Here's how the part is built. I have some questions about the finished solid (model axes, mm). Face numbers are marked on the shaded views. A direction names the side the tool comes from. Round coordinates to 2 decimals unless told otherwise and drop trailing zeros. Write each loop counter-clockwise with the first axis right and the second up, starting at its lowest first coordinate (ties: lowest second). Pieces come first, ordered by that corner, then holes. Notation, with made-up numbers: (-37.75, -1.5) -> (-14.75, -1.5) arc R29 ccw to (-14.75, 18.5) -> close; hole circle Ø9 at (68, 35). An arc over 180 degrees is marked (long way). Put each result on its own line as item: value. Start each with the question number.
1. Suppose I cut it at B-B (z = 25). Count the separate pieces of the cut face and the enclosed holes in it, then the cut area to 3 significant figures.
2. Suppose I cut it at A-A (y = 47.5). Please give me the cut outline in (x, z).
3. We'd pull the mould along Y, two halves only. Please class the marked faces 1, 2, 3 and 4: +Y half, -Y half, draft (parallel to the pull), parting line (faces both ways), or undercut.
4. I need wall thicknesses on probe 1 along Y at (x, z) = (0, 21); probe 2 along Y at (x, z) = (0, -3); probe 3 along Z at (x, y) = (-28, 38). Which ranges of each line are inside material? Lowest first, please. Write a range as from..to.
5. For pin 1 (8 mm diameter, centred on x = 25, y = 65, fed in from -Z); pin 2 (3 mm diameter, centred on y = 13, z = 49.5, fed in from +X); pin 3 (7 mm diameter, centred on x = 0, y = 0, fed in from -Z); pin 4 (6 mm diameter, centred on x = -58, y = 32, fed in from -Z), each with a flat end and sliding along its axis, tell me the tip position at first contact or that it passes through.
6. Suppose I cut it at D-D (y = 31). Please give me the cut outline in (x, z), then the cut area to 3 significant figures.
7. Which directions (+Z, -Z, +X, -X, +Y, -Y) give clear straight access to the entire face, cutting with the end or side of a thin tool? Please do the marked faces 5, 6, 7 and 8.
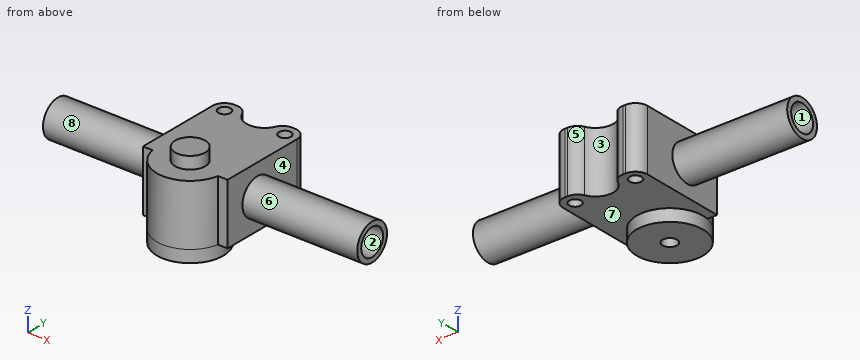
```python
from build123d import *

# Parameters (mm, degrees)
SKETCH1_R           = 5
BOSS_EXTRUDE2_DEPTH = 50
SHELL2_START        = 5
SHELL2_DEPTH        = 40
SKETCH3_R           = 15
CUT_EXTRUDE1_DEPTH  = 5
BOSS_EXTRUDE3_START = 10
SKETCH4_R           = 27.5
SKETCH4_R_2         = 6
BOSS_EXTRUDE3_DEPTH = 10
SKETCH5_R           = 15
SKETCH5_R_2         = 11
BOSS_EXTRUDE4_DEPTH = 95
CUT_EXTRUDE2_START  = -80
SKETCH5_2_R         = 11
CUT_EXTRUDE2_DEPTH  = 80
BOSS_EXTRUDE5_START = -165
SKETCH5_3_R         = 15
SKETCH5_3_R_2       = 11
BOSS_EXTRUDE5_DEPTH = 95
SKETCH6_R           = 12.5
SKETCH6_R_2         = 6
BOSS_EXTRUDE6_DEPTH = 5
CUT_EXTRUDE3_START  = -5
SKETCH6_2_R         = 6
CUT_EXTRUDE3_DEPTH  = 5
BOSS_EXTRUDE7_START = -38
SKETCH6_3_R         = 12.5
SKETCH6_3_R_2       = 6
BOSS_EXTRUDE7_DEPTH = 38
SKETCH6_4_R         = 12.5
SKETCH6_4_R_2       = 6
BOSS_EXTRUDE8_DEPTH = 10


# Read off the part's stored shape, not the designer's step: Shell2
with BuildPart() as part:
    # Sketch1 → Boss-Extrude2 (new body)
    with BuildSketch(Plane.XY):
        with BuildLine():
            Line((22.912878475, 75), (25, 75))
            ThreePointArc((25, 75), (32.071067812, 72.071067812), (35, 65))
            Line((35, 65), (35, -5))
            Line((35, -5), (27.041634566, -5))
            ThreePointArc((27.041634566, -5), (0, -27.5), (-27.041634566, -5))
            Line((-27.041634566, -5), (-35, -5))
            Line((-35, -5), (-35, 65))
            ThreePointArc((-35, 65), (-32.071067812, 72.071067812), (-25, 75))
            Line((-25, 75), (-22.912878475, 75))
            ThreePointArc((-22.912878475, 75), (-17.4356529, 73.366600265), (-13.747727085, 69))
            ThreePointArc((-13.747727085, 69), (0, 60), (13.747727085, 69))
            ThreePointArc((13.747727085, 69), (17.4356529, 73.366600265), (22.912878475, 75))
        make_face()
        with Locations((-25, 65)):
            Circle(SKETCH1_R, mode=Mode.SUBTRACT)
        with Locations((25, 65)):
            Circle(SKETCH1_R, mode=Mode.SUBTRACT)
    extrude(amount=BOSS_EXTRUDE2_DEPTH)

    # Shell2 outline → Shell2 (cut)
    with BuildSketch(Plane.XY.offset(SHELL2_START)):
        with BuildLine():
            Line((30, 0), (30, 56.339745962))
            ThreePointArc((30, 56.339745962), (21.260998255, 55.725310466), (15.391593697, 62.228984243))
            ThreePointArc((15.391593697, 62.228984243), (0, 55), (-15.391593697, 62.228984243))
            ThreePointArc((-15.391593697, 62.228984243), (-21.260998255, 55.725310466), (-30, 56.339745962))
            Line((-30, 56.339745962), (-30, 0))
            Line((-30, 0), (-22.5, 0))
            ThreePointArc((-22.5, 0), (0, -22.5), (22.5, 0))
            Line((22.5, 0), (30, 0))
        make_face()
    extrude(amount=SHELL2_DEPTH, mode=Mode.SUBTRACT)

    # Sketch3 → Cut-Extrude1 (cut)
    with BuildSketch(Plane(origin=(0, 0, 0), x_dir=(-1, 0, 0), z_dir=(0, 0, -1))):
        Circle(SKETCH3_R)
    extrude(amount=-CUT_EXTRUDE1_DEPTH, mode=Mode.SUBTRACT)

    # Sketch4 → Boss-Extrude3 (add)
    with BuildSketch(Plane(origin=(0, 0, 0), x_dir=(-1, 0, 0), z_dir=(0, 0, -1)).offset(BOSS_EXTRUDE3_START)):
        Circle(SKETCH4_R)
        Circle(SKETCH4_R_2, mode=Mode.SUBTRACT)
    extrude(amount=-BOSS_EXTRUDE3_DEPTH)

    # Sketch5 → Boss-Extrude4 (add)
    with BuildSketch(Plane(origin=(35, 0, 0), x_dir=(0, 0, -1), z_dir=(1, 0, 0))):
        with Locations(Location((-25, 25, 0), (0, 0, 270))):
            Circle(SKETCH5_R)
        with Locations(Location((-25, 25, 0), (0, 0, 90))):
            Circle(SKETCH5_R_2, mode=Mode.SUBTRACT)
    extrude(amount=BOSS_EXTRUDE4_DEPTH)

    # Sketch5<2> → Cut-Extrude2 (cut)
    with BuildSketch(Plane(origin=(35, 0, 0), x_dir=(0, 0, -1), z_dir=(1, 0, 0)).offset(CUT_EXTRUDE2_START)):
        with Locations(Location((-25, 25, 0), (0, 0, 270))):
            Circle(SKETCH5_2_R)
    extrude(amount=CUT_EXTRUDE2_DEPTH, mode=Mode.SUBTRACT)

    # Sketch5<3> → Boss-Extrude5 (add)
    with BuildSketch(Plane(origin=(35, 0, 0), x_dir=(0, 0, -1), z_dir=(1, 0, 0)).offset(BOSS_EXTRUDE5_START)):
        with Locations(Location((-25, 25, 0), (0, 0, 270))):
            Circle(SKETCH5_3_R)
        with Locations(Location((-25, 25, 0), (0, 0, 270))):
            Circle(SKETCH5_3_R_2, mode=Mode.SUBTRACT)
    extrude(amount=BOSS_EXTRUDE5_DEPTH)

    # Sketch6 → Boss-Extrude6 (add)
    with BuildSketch(Plane.XY.offset(50)):
        with Locations(Location((0, 0, 0), (0, 0, 180))):
            Circle(SKETCH6_R)
        with Locations(Location((0, 0, 0), (0, 0, 180))):
            Circle(SKETCH6_R_2, mode=Mode.SUBTRACT)
    extrude(amount=BOSS_EXTRUDE6_DEPTH)

    # Sketch6<2> → Cut-Extrude3 (cut)
    with BuildSketch(Plane.XY.offset(50).offset(CUT_EXTRUDE3_START)):
        with Locations(Location((0, 0, 0), (0, 0, 180))):
            Circle(SKETCH6_2_R)
    extrude(amount=CUT_EXTRUDE3_DEPTH, mode=Mode.SUBTRACT)

    # Sketch6<3> → Boss-Extrude7 (add)
    with BuildSketch(Plane.XY.offset(50).offset(BOSS_EXTRUDE7_START)):
        with Locations(Location((0, 0, 0), (0, 0, 180))):
            Circle(SKETCH6_3_R)
        with Locations(Location((0, 0, 0), (0, 0, 180))):
            Circle(SKETCH6_3_R_2, mode=Mode.SUBTRACT)
    extrude(amount=BOSS_EXTRUDE7_DEPTH)

    # Sketch6<4> → Boss-Extrude8 (add)
    # profile 1 of 2: a face of its own
    with BuildSketch(Plane.XY.offset(50)):
        with Locations(Location((0, 0, 0), (0, 0, 180))):
            Circle(SKETCH6_4_R)
        Circle(SKETCH6_4_R_2, mode=Mode.SUBTRACT)
    # profile 2 of 2: a face of its own
    with BuildSketch(Plane.XY.offset(50)):
        Circle(SKETCH6_4_R_2)
    extrude(amount=BOSS_EXTRUDE8_DEPTH)


solid = part.part
```
Verdict:
1. separate pieces: 3
1. enclosed holes: 3
1. area: 3,410 mm^2
2. outline: (-35, 0) -> (35, 0) -> (35, 50) -> (-35, 50) -> close; hole (-30, 5) -> (30, 5) -> (30, 45) -> (-30, 45) -> close
3. face 1: undercut
3. face 2: undercut
3. face 3: +Y half
3. face 4: draft
4. probe 1: y = -27.5..-22.5, -12.5..-6, 6..12.5, 55..60
4. probe 2: y = -27.5..-6, 6..27.5
4. probe 3: z = 0..5, 45..50
5. pin 1: passes through
5. pin 2: stops at x = 35
5. pin 3: stops at z = 50
5. pin 4: stops at z = 10.54
6. outline: (-130, 11.25) -> (-35, 11.25) -> (-35, 0) -> (35, 0) -> (35, 11.25) -> (130, 11.25) -> (130, 15.78) -> (30, 15.78) -> (30, 5) -> (-30, 5) -> (-30, 15.78) -> (-130, 15.78) -> close; (-130, 34.22) -> (-30, 34.22) -> (-30, 45) -> (30, 45) -> (30, 34.22) -> (130, 34.22) -> (130, 38.75) -> (35, 38.75) -> (35, 50) -> (-35, 50) -> (-35, 38.75) -> (-130, 38.75) -> close
6. area: 2,640 mm^2
7. face 5: +Z, -Z, +Y
7. face 6: +X
7. face 7: -Z, +Y
7. face 8: -X
